```python
from build123d import *

# Parameters (mm, degrees)
EXTRUDE1_DEPTH     = 2.413
SKETCH4_R          = 3.5687
EXTRUDE3_DEPTH     = 0.762
SKETCH6_R          = 3.175
CUT_EXTRUDE1_DEPTH = 4.175


with BuildPart() as part:
    # Sketch1 → Extrude1 (new body)
    with BuildSketch(Plane.XY):
        with BuildLine():
            Line((111.27866266, 131.559165896), (125.42646266, 131.559165896))
            ThreePointArc((125.42646266, 131.559165896), (131.05256266, 125.933065896), (125.42646266, 120.306965896))
            Line((125.42646266, 120.306965896), (111.27866266, 120.306965896))
            ThreePointArc((111.27866266, 120.306965896), (105.65256266, 125.933065896), (111.27866266, 131.559165896))
        make_face()
    extrude(amount=EXTRUDE1_DEPTH)

    # Sketch4 → Extrude3 (add)
    with BuildSketch(Plane.XY.offset(2.413)):
        with Locations((118.35256266, 125.933065896)):
            Circle(SKETCH4_R)
    extrude(amount=EXTRUDE3_DEPTH)

    # Sketch6 → Cut-Extrude1 (cut, through all)
    with BuildSketch(Plane(origin=(0, 0, 0), x_dir=(-1, 0, 0), z_dir=(0, 0, -1))):
        with Locations((-118.35256266, 125.933065896)):
            Circle(SKETCH6_R)
    extrude(amount=-CUT_EXTRUDE1_DEPTH, mode=Mode.SUBTRACT)


solid = part.part
```
Could you check a few things on this model? Use its own coordinates, in mm. A direction names the side the tool comes from. Give positions to 0.01 mm unless a question says otherwise; leave off trailing zeros. Order: outer loops, then holes, each group sorted by start corner. A loop starts at its lowest first (then second) coordinate and runs counter-clockwise, first axis right, second up.
Q1. We'd pull the mould along Y, two halves only. Please class faces 3 (the flat face through (118, 120.307, 1)), 4 (the flat face through (121.4, 127.3, 0)), 5 (the cylindrical face through (115.42, 124.72, 1.57)): +Y half, -Y half, draft (parallel to the pull), parting line (faces both ways), or undercut.
Q2. Suppose I cut it at C-C, the plane z = 0.6. Write out the boundary of the cut face in (x, y) (3 decimals).
Q3. Suppose I cut it at A-A, the plane y = 128.5. Write out the boundary of the cut face in (x, z) (3 decimals), and give its area (3 significant figures).
Q4. I'm going to push flat-ended pins straight in: P1, Ø1, axis at y = 129.5, z = 1.5, coming from the +X side; P2, Ø1.5, axis at y = 130, z = 2.5, coming from the +X side; P3, Ø1.5, axis at x = 109, y = 123.5, coming from the +Z side. Where does each tip first touch, or does it pass through?
Q5. If I drill on line 1 along Y through (x, z) = (118.25, 1.6); line 2 along Z through (x, y) = (114.75, 121.25); line 3 along X through (y, z) = (125.75, 0.4), over which ranges is the centre line in solid material (lowest first)?
Q6. Suppose I cut it at B-B, the plane x = 116. Write out the boundary of the cut face in (y, z) (3 decimals), and give its area (3 significant figures).
Q7. For faces 1 (the cylindrical face through (117.89, 129.47, 2.79)), 2 (the flat face through (115, 126, 3.175)), which set-ups out of +Z, -Z, +X, -X, +Y, -Y let a thin tool reach every point of the face, with its end or its side?
Q8. Suppose I cut it at D-D, the plane x = 124.5. Write out the boundary of the cut face in (y, z), and give its area (3 significant figures).
Solution:
1. face 3: -Y half
1. face 4: draft
1. face 5: undercut
2. outline: (111.279, 120.307) - (125.426, 120.307) arc R5.626 ccw to (125.426, 131.559) - (111.279, 131.559) arc R5.626 ccw to start; hole circle Ø6.35 at (118.353, 125.933)
3. outline: (106.272, 0) - (116.484, 0) - (116.484, 3.175) - (115.873, 3.175) - (115.873, 2.413) - (106.272, 2.413) - close; (120.221, 0) - (130.433, 0) - (130.433, 2.413) - (120.832, 2.413) - (120.832, 3.175) - (120.221, 3.175) - close
3. area: 50.2 mm2
4. P1: stops at x = 130.14
4. P2: stops at x = 129.97
4. P3: stops at z = 2.41
5. line 1: y = 120.31 to 122.76, 129.11 to 131.56
5. line 2: z = 0 to 2.41
5. line 3: x = 105.66 to 115.18, 121.52 to 131.05
6. outline: (120.307, 0) - (123.801, 0) - (123.801, 3.175) - (123.25, 3.175) - (123.25, 2.413) - (120.307, 2.413) - close; (128.065, 0) - (131.559, 0) - (131.559, 2.413) - (128.617, 2.413) - (128.617, 3.175) - (128.065, 3.175) - close
6. area: 17.7 mm2
7. face 1: +Z
7. face 2: +Z, +X, -X, +Y, -Y
8. outline: (120.31, 0) - (131.56, 0) - (131.56, 2.41) - (120.31, 2.41) - close
8. area: 27.2 mm2
